Design review of the part built by this model. Coordinates are the model's own, in mm. Coordinates: 2 decimals unless noted, no trailing zeros. Write each loop counter-clockwise with the first axis right and the second up, starting at its lowest first coordinate (ties: lowest second). Pieces come first, ordered by that corner, then holes. Notation, with made-up numbers: M 75,9.25 L 120,9.25 A27 ccw 120,44.25 Z; hole C -20,89.25 d5. An arc over 180 degrees is marked long. Write item = value, one per line.
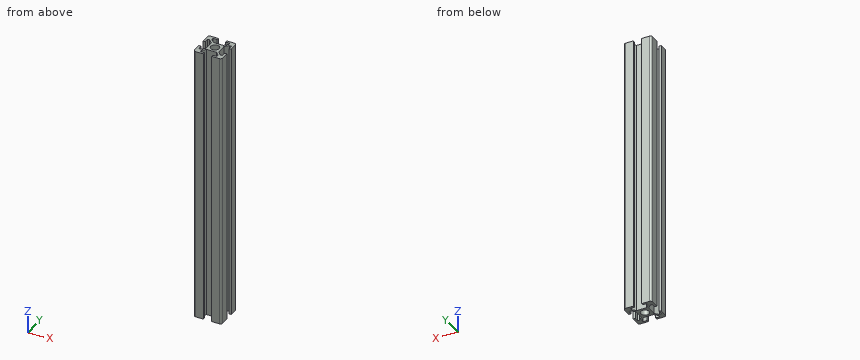
```python
from build123d import *

# Parameters (mm, degrees)
F0_R     = 3
F1_DEPTH = 200


with BuildPart() as f1:
    # F0 (on Top) → F1 (new body)
    with BuildSketch(Plane.XY):
        with BuildLine():
            ThreePointArc((0, 1.5), (0.43934, 0.43934), (1.5, 0))
            Line((1.5, 0), (7, 0))
            Line((7, 0), (7, 1.5))
            Line((7, 1.5), (4, 1.5))
            Line((4, 1.5), (4, 3))
            Line((4, 3), (6.5, 5.5))
            Line((6.5, 5.5), (10, 5.5))
            Line((10, 5.5), (13.5, 5.5))
            Line((13.5, 5.5), (16, 3))
            Line((16, 3), (16, 1.5))
            Line((16, 1.5), (13, 1.5))
            Line((13, 1.5), (13, 0))
            Line((13, 0), (18.5, 0))
            ThreePointArc((18.5, 0), (19.56066, 0.43934), (20, 1.5))
            Line((20, 1.5), (20, 7))
            Line((20, 7), (18.5, 7))
            Line((18.5, 7), (18.5, 4))
            Line((18.5, 4), (17, 4))
            Line((17, 4), (14.5, 6.5))
            Line((14.5, 6.5), (14.5, 10))
            Line((14.5, 10), (14.5, 13.5))
            Line((14.5, 13.5), (17, 16))
            Line((17, 16), (18.5, 16))
            Line((18.5, 16), (18.5, 13))
            Line((18.5, 13), (20, 13))
            Line((20, 13), (20, 18.5))
            ThreePointArc((20, 18.5), (19.56066, 19.56066), (18.5, 20))
            Line((18.5, 20), (13, 20))
            Line((13, 20), (13, 18.5))
            Line((13, 18.5), (16, 18.5))
            Line((16, 18.5), (16, 17))
            Line((16, 17), (13.5, 14.5))
            Line((13.5, 14.5), (10, 14.5))
            Line((10, 14.5), (6.5, 14.5))
            Line((6.5, 14.5), (4, 17))
            Line((4, 17), (4, 18.5))
            Line((4, 18.5), (7, 18.5))
            Line((7, 18.5), (7, 20))
            Line((7, 20), (1.5, 20))
            ThreePointArc((1.5, 20), (0.43934, 19.56066), (0, 18.5))
            Line((0, 18.5), (0, 13))
            Line((0, 13), (1.5, 13))
            Line((1.5, 13), (1.5, 16))
            Line((1.5, 16), (3, 16))
            Line((3, 16), (5.5, 13.5))
            Line((5.5, 13.5), (5.5, 10))
            Line((5.5, 10), (5.5, 6.5))
            Line((5.5, 6.5), (3, 4))
            Line((3, 4), (1.5, 4))
            Line((1.5, 4), (1.5, 7))
            Line((1.5, 7), (0, 7))
            Line((0, 7), (0, 1.5))
        make_face()
        with Locations((10, 10)):
            Circle(F0_R, mode=Mode.SUBTRACT)
    extrude(amount=F1_DEPTH)


solid = f1.part
```
Q1. For P1, Ø1.2, axis at y = 0.5, z = 132.5, coming from the +X side; P2, Ø0.8, axis at y = 19, z = 143, coming from the -X side; P3, Ø1.2, axis at x = 19.5, z = 103, coming from the -Y side, all flat-tipped, find the tip position at first contact; note any pin that passes through.
Check result:
P1 = 19.95
P2 = 0
P3 = 0.05
Q2. Consider section A-A, the plane y = 10. State the section outline as (x, z) points, and give its area (3 significant figures).
Check result:
outline = M 5.5,0 L 7,0 L 7,200 L 5.5,200 Z; M 13,0 L 14.5,0 L 14.5,200 L 13,200 Z
area = 600 mm²
Q3. Wall thickness on line 1 (X direction, y = 13.25, z = 94); line 2 (X direction, y = 3, z = 105): over which ranges is each line inside the solid? List them lowest first.
Check result:
line_1 = 0 to 1.5, 5.5 to 14.5, 18.5 to 20
line_2 = 0 to 4, 16 to 20
